Verification items for the finished model (mm, model axes). A direction names the side the tool comes from. Coordinates: 2 decimals unless noted, no trailing zeros. Order: outer loops, then holes, each group sorted by start corner. A loop starts at its lowest first (then second) coordinate and runs counter-clockwise, first axis right, second up. Notation, with made-up numbers: M -9.5,39 L 16.5,39 A10 ccw 16.5,45 Z; hole C 63.25,31.25 d9. An arc over 180 degrees is marked long. Return JSON: item names as keys, results as strings. Group by question number.
Q1. Section check A-A, the plane z = 25.4. Enter the section's corners in (x, y) (1 decimal).
Q2. Thickness scan on probe 1 along X at (y, z) = (-4.25, 7); probe 2 along Z at (x, y) = (-52, -2); probe 3 along Y at (x, z) = (-55, 44.5) (1 decimal). Record the ranges inside material, lowest first.
Q3. Access from +Z, -Z, +X, -X, +Y, -Y to the whole of each face (thin tool, end or side, straight path). Record for faces 1 (the face through (-26, -7.938, 58)), 2 (the face through (0, -8.1, 54.8)), 3 (the face through (0, -4, 25)), 4 (the face through (-58, -7.938, 25)).
Q4. Section check D-D, the plane z = 43. Enter the section's corners in (x, y) (1 decimal).
Q5. Section check C-C, the plane y = -5.5. Enter the section's corners in (x, z).
Q6. Go/stop test with flat-tipped pins: pin 1 Ø5 at (x, y) = (-13.5, -5) entering from -Z; pin 2 Ø1.9 at (y, z) = (-2.5, 25) entering from -X; pin 3 Ø5 at (x, z) = (9, 18) entering from +Y; pin 4 Ø18.5 at (x, z) = (-25.4, 25.4) entering from +Y. Record where each tip stops, or that it passes through.
Q7. Section check B-B, the plane x = -25.4. Enter the section's corners in (y, z) (1 decimal).
Q8. Mould release check, pull along Z, two halves, no side actions. Record for faces 5 (the face through (-22.907, 0.805, 14.173)), 6 (the face through (-26, -9, 63.5)), 7 (the face through (1.588, -4, 25)): pulls with the +Z half, pulls with the -Z half, needs draft (parallel to the pull), parting line crosses it, or undercut.
from build123d import *

# Parameters (mm, degrees)
SKETCH6_W                      = 50.8
SKETCH6_H                      = 1.5875
BASE_FLANGE1_DEPTH             = 50.8
EDGE_FLANGE1_STRIP_W           = 7.8232
EDGE_FLANGE1_STRIP_H           = 1.5875
EDGE_FLANGE1_STRIP_CUT_DEPTH   = 50.8
EDGE_FLANGE1_DEPTH             = 50.8
SKETCH16_R                     = 11.5
CUT_EXTRUDE1_DEPTH             = 74.592226364
EDGE_FLANGE4_STRIP_W           = 7.8232
EDGE_FLANGE4_STRIP_H           = 1.5875
EDGE_FLANGE4_STRIP_CUT_DEPTH   = 50.0634
EDGE_FLANGE4_STRIP_2_W         = 7.8232
EDGE_FLANGE4_STRIP_2_H         = 1.5875
EDGE_FLANGE4_STRIP_CUT_2_DEPTH = 50.0634
EDGE_FLANGE4_DEPTH             = 50.0634
EDGE_FLANGE4_BEND_DEPTH        = 50.0634
EDGE_FLANGE5_STRIP_W           = 7.8232
EDGE_FLANGE5_STRIP_H           = 1.5875
EDGE_FLANGE5_STRIP_CUT_DEPTH   = 50.0634
EDGE_FLANGE5_STRIP_2_W         = 7.8232
EDGE_FLANGE5_STRIP_2_H         = 1.5875
EDGE_FLANGE5_STRIP_CUT_2_DEPTH = 50.0634
EDGE_FLANGE5_DEPTH             = 50.0634
EDGE_FLANGE5_BEND_DEPTH        = 50.0634
EDGE_FLANGE6_STRIP_W           = 7.8232
EDGE_FLANGE6_STRIP_H           = 1.5875
EDGE_FLANGE6_STRIP_CUT_DEPTH   = 50.8
EDGE_FLANGE6_DEPTH             = 50.8


# Sheet-metal steps are written as plain solids
with BuildPart() as part:
    # Sketch6 → Base-Flange1 (new body)
    with BuildSketch(Plane.XY):
        with Locations((-25.4, 0.79375)):
            Rectangle(SKETCH6_W, SKETCH6_H)
    extrude(amount=BASE_FLANGE1_DEPTH)

    # Edge-Flange1 strip (across the edge) → Edge-Flange1 strip cut (cut)
    with BuildSketch(Plane(origin=(0, 0, 50.8), x_dir=(0, 0, -1), z_dir=(-1, 0, 0))):
        with Locations((-3.175, -0.79375)):
            Rectangle(EDGE_FLANGE1_STRIP_W, EDGE_FLANGE1_STRIP_H)
    extrude(amount=EDGE_FLANGE1_STRIP_CUT_DEPTH, mode=Mode.SUBTRACT)

    # Edge-Flange1 section (across the edge) → Edge-Flange1 (add)
    with BuildSketch(Plane(origin=(0, 0, 50.8), x_dir=(0, 0, -1), z_dir=(-1, 0, 0))):
        with BuildLine():
            Line((-1.5875, 0.7366), (-1.5875, 7.9375))
            Line((-1.5875, 7.9375), (0, 7.9375))
            Line((0, 7.9375), (0, 0.7366))
            ThreePointArc((0, 0.7366), (0.215745145, 0.215745145), (0.7366, 0))
            Line((0.7366, 0), (0.7366, -1.5875))
            ThreePointArc((0.7366, -1.5875), (-0.90678687, -0.90678687), (-1.5875, 0.7366))
        make_face()
    extrude(amount=EDGE_FLANGE1_DEPTH)

    # Sketch16 → Cut-Extrude1 (cut, through all)
    with BuildSketch(Plane(origin=(0, 1.5875, 0), x_dir=(1, 0, 0), z_dir=(0, 1, 0))):
        with Locations(Location((-25.4, -25.4, 0), (0, 0, 180))):
            Circle(SKETCH16_R)
    extrude(amount=-CUT_EXTRUDE1_DEPTH, mode=Mode.SUBTRACT)

    # Edge-Flange4 strip (across the edge) → Edge-Flange4 strip cut (cut)
    with BuildSketch(Plane(origin=(0, 0, 0), x_dir=(-1, 0, 0), z_dir=(0, 0, 1))):
        with Locations((-3.175, -0.79375)):
            Rectangle(EDGE_FLANGE4_STRIP_W, EDGE_FLANGE4_STRIP_H)
    extrude(amount=EDGE_FLANGE4_STRIP_CUT_DEPTH, mode=Mode.SUBTRACT)

    # Edge-Flange4 strip 2 (across the edge) → Edge-Flange4 strip cut 2 (cut)
    with BuildSketch(Plane(origin=(-50.8, 0, 50.0634), x_dir=(1, 0, 0), z_dir=(0, 0, -1))):
        with Locations((-3.175, -0.79375)):
            Rectangle(EDGE_FLANGE4_STRIP_2_W, EDGE_FLANGE4_STRIP_2_H)
    extrude(amount=EDGE_FLANGE4_STRIP_CUT_2_DEPTH, mode=Mode.SUBTRACT)

    # Edge-Flange4 section (across the edge) → Edge-Flange4 (add)
    with BuildSketch(Plane(origin=(0, 0, 0), x_dir=(-1, 0, 0), z_dir=(0, 0, 1))):
        with BuildLine():
            Line((-1.5875, 0.7366), (-1.5875, 7.9375))
            Line((-1.5875, 7.9375), (0, 7.9375))
            Line((0, 7.9375), (0, 0.7366))
            ThreePointArc((0, 0.7366), (0.215745145, 0.215745145), (0.7366, 0))
            Line((0.7366, 0), (0.7366, -1.5875))
            ThreePointArc((0.7366, -1.5875), (-0.90678687, -0.90678687), (-1.5875, 0.7366))
        make_face()
    extrude(amount=EDGE_FLANGE4_DEPTH)

    # Edge-Flange4 section 2 (across the edge) → Edge-Flange4 bend (add)
    with BuildSketch(Plane(origin=(-50.8, 0, 50.0634), x_dir=(1, 0, 0), z_dir=(0, 0, -1))):
        with BuildLine():
            Line((-1.5875, 0.7366), (-1.5875, 7.9375))
            Line((-1.5875, 7.9375), (0, 7.9375))
            Line((0, 7.9375), (0, 0.7366))
            ThreePointArc((0, 0.7366), (0.215745145, 0.215745145), (0.7366, 0))
            Line((0.7366, 0), (0.7366, -1.5875))
            ThreePointArc((0.7366, -1.5875), (-0.90678687, -0.90678687), (-1.5875, 0.7366))
        make_face()
    extrude(amount=EDGE_FLANGE4_BEND_DEPTH)

    # Edge-Flange5 strip (across the edge) → Edge-Flange5 strip cut (cut)
    with BuildSketch(Plane(origin=(1.5875, -7.9375, 50.0634), x_dir=(0, 1, 0), z_dir=(0, 0, -1))):
        with Locations((-3.175, -0.79375)):
            Rectangle(EDGE_FLANGE5_STRIP_W, EDGE_FLANGE5_STRIP_H)
    extrude(amount=EDGE_FLANGE5_STRIP_CUT_DEPTH, mode=Mode.SUBTRACT)

    # Edge-Flange5 strip 2 (across the edge) → Edge-Flange5 strip cut 2 (cut)
    with BuildSketch(Plane(origin=(-52.3875, -7.9375, 0), x_dir=(0, 1, 0), z_dir=(0, 0, 1))):
        with Locations((-3.175, -0.79375)):
            Rectangle(EDGE_FLANGE5_STRIP_2_W, EDGE_FLANGE5_STRIP_2_H)
    extrude(amount=EDGE_FLANGE5_STRIP_CUT_2_DEPTH, mode=Mode.SUBTRACT)

    # Edge-Flange5 section (across the edge) → Edge-Flange5 (add)
    with BuildSketch(Plane(origin=(1.5875, -7.9375, 50.0634), x_dir=(0, 1, 0), z_dir=(0, 0, -1))):
        with BuildLine():
            Line((-1.5875, 0.7366), (-1.5875, 11.1125))
            Line((-1.5875, 11.1125), (0, 11.1125))
            Line((0, 11.1125), (0, 0.7366))
            ThreePointArc((0, 0.7366), (0.215745145, 0.215745145), (0.7366, 0))
            Line((0.7366, 0), (0.7366, -1.5875))
            ThreePointArc((0.7366, -1.5875), (-0.90678687, -0.90678687), (-1.5875, 0.7366))
        make_face()
    extrude(amount=EDGE_FLANGE5_DEPTH)

    # Edge-Flange5 section 2 (across the edge) → Edge-Flange5 bend (add)
    with BuildSketch(Plane(origin=(-52.3875, -7.9375, 0), x_dir=(0, 1, 0), z_dir=(0, 0, 1))):
        with BuildLine():
            Line((-1.5875, 0.7366), (-1.5875, 11.1125))
            Line((-1.5875, 11.1125), (0, 11.1125))
            Line((0, 11.1125), (0, 0.7366))
            ThreePointArc((0, 0.7366), (0.215745145, 0.215745145), (0.7366, 0))
            Line((0.7366, 0), (0.7366, -1.5875))
            ThreePointArc((0.7366, -1.5875), (-0.90678687, -0.90678687), (-1.5875, 0.7366))
        make_face()
    extrude(amount=EDGE_FLANGE5_BEND_DEPTH)

    # Edge-Flange6 strip (across the edge) → Edge-Flange6 strip cut (cut)
    with BuildSketch(Plane(origin=(-50.8, -7.9375, 52.3875), x_dir=(0, 1, 0), z_dir=(1, 0, 0))):
        with Locations((-3.175, -0.79375)):
            Rectangle(EDGE_FLANGE6_STRIP_W, EDGE_FLANGE6_STRIP_H)
    extrude(amount=EDGE_FLANGE6_STRIP_CUT_DEPTH, mode=Mode.SUBTRACT)

    # Edge-Flange6 section (across the edge) → Edge-Flange6 (add)
    with BuildSketch(Plane(origin=(-50.8, -7.9375, 52.3875), x_dir=(0, 1, 0), z_dir=(1, 0, 0))):
        with BuildLine():
            Line((-1.5875, 0.7366), (-1.5875, 11.1125))
            Line((-1.5875, 11.1125), (0, 11.1125))
            Line((0, 11.1125), (0, 0.7366))
            ThreePointArc((0, 0.7366), (0.215745145, 0.215745145), (0.7366, 0))
            Line((0.7366, 0), (0.7366, -1.5875))
            ThreePointArc((0.7366, -1.5875), (-0.90678687, -0.90678687), (-1.5875, 0.7366))
        make_face()
    extrude(amount=EDGE_FLANGE6_DEPTH)


solid = part.part
Numbers:
{
 "1": {"outline": "M -63.5,-9.5 L -53.1,-9.5 A2.3 ccw -50.8,-7.2 L -50.8,-0.7 A0.7 cw -50.1,0 L -36.9,0 L -36.9,1.6 L -50.1,1.6 A2.3 ccw -52.4,-0.7 L -52.4,-7.2 A0.7 cw -53.1,-7.9 L -63.5,-7.9 Z; M -13.9,0 L -0.7,0 A0.7 cw 0,-0.7 L 0,-7.2 A2.3 ccw 2.3,-9.5 L 12.7,-9.5 L 12.7,-7.9 L 2.3,-7.9 A0.7 cw 1.6,-7.2 L 1.6,-0.7 A2.3 ccw -0.7,1.6 L -13.9,1.6 Z"},
 "2": {"probe 1": "x = -52.39 to -50.8, 0 to 1.59", "probe 2": "z = 0 to 50.06", "probe 3": "y = -9.5 to -7.9"},
 "3": {"face 1": "+Z, +X, -X, +Y", "face 2": "+Z, +X, +Y, -Y", "face 3": "-Z, -Y", "face 4": "+Z, -Z, -X, +Y"},
 "4": {"outline": "M -63.5,-9.5 L -53.1,-9.5 A2.3 ccw -50.8,-7.2 L -50.8,-0.7 A0.7 cw -50.1,0 L -0.7,0 A0.7 cw 0,-0.7 L 0,-7.2 A2.3 ccw 2.3,-9.5 L 12.7,-9.5 L 12.7,-7.9 L 2.3,-7.9 A0.7 cw 1.6,-7.2 L 1.6,-0.7 A2.3 ccw -0.7,1.6 L -50.1,1.6 A2.3 ccw -52.4,-0.7 L -52.4,-7.2 A0.7 cw -53.1,-7.9 L -63.5,-7.9 Z"},
 "5": {"outline": "M -52.39,0 L -50.8,0 L -50.8,50.06 L -52.39,50.06 Z; M -50.8,50.8 L 0,50.8 L 0,52.39 L -50.8,52.39 Z; M 0,0 L 1.59,0 L 1.59,50.06 L 0,50.06 Z"},
 "6": {"pin 1": "stops at z = 50.8", "pin 2": "stops at x = -52.39", "pin 3": "stops at y = -7.94", "pin 4": "passes through"},
 "7": {"outline": "M -9.5,53.1 A2.3 ccw -7.2,50.8 L -0.7,50.8 A0.7 cw 0,50.1 L 0,36.9 L 1.6,36.9 L 1.6,50.1 A2.3 ccw -0.7,52.4 L -7.2,52.4 A0.7 cw -7.9,53.1 L -7.9,63.5 L -9.5,63.5 Z; M 0,0 L 1.6,0 L 1.6,13.9 L 0,13.9 Z"},
 "8": {"face 5": "undercut", "face 6": "pulls with the +Z half", "face 7": "needs draft"}
}
